Verification items for the finished model (mm, model axes). A direction names the side the tool comes from. Round coordinates to 2 decimals unless told otherwise and drop trailing zeros. Order: outer loops, then holes, each group sorted by start corner. A loop starts at its lowest first (then second) coordinate and runs counter-clockwise, first axis right, second up. Notation, with made-up numbers: M 55.25,84 L 96.25,84 A14 cw 96.25,97 Z; hole C 9,20.25 d6. An arc over 180 degrees is marked long. Answer as a JSON object with one key per item and string values. Group by question number.
```python
from build123d import *

# Parameters (mm, degrees)
ESQUISSE1_R                  = 7.5
BOSS_EXTRU_1_DEPTH           = 10
ESQUISSE1_5_R                = 14
ENL_V_MAT_EXTRU_1_DEPTH      = 2
ENL_V_MAT_EXTRU_1_DEPTH_BACK = 10
BOSS_EXTRU_2_DEPTH           = 45
ENL_V_MAT_EXTRU_2_DEPTH      = 11
ENL_V_MAT_EXTRU_2_DEPTH_BACK = 21


with BuildPart() as part:
    # Esquisse1 → Boss.-Extru.1 (new body, symmetric)
    with BuildSketch(Plane.XY):
        with BuildLine():
            Line((-634.508066615, 20.5), (-595.008671928, 20.5))
            Line((-595.008671928, 20.5), (-595.008671928, -24.5))
            Line((-595.008671928, -24.5), (-634.508066615, -24.5))
            ThreePointArc((-634.508066615, -24.5), (-657.008066615, -2), (-634.508066615, 20.5))
        make_face()
        with Locations((-634.508066615, -2)):
            Circle(ESQUISSE1_R, mode=Mode.SUBTRACT)
    extrude(amount=BOSS_EXTRU_1_DEPTH, both=True)

    # Esquisse1_5 → Enl_v. mat.-Extru.1 (cut, two sides)
    with BuildSketch(Plane.XY) as enl_v_mat_extru_1_sk:
        with Locations((-634.508066615, -2)):
            Circle(ESQUISSE1_5_R)
    extrude(amount=ENL_V_MAT_EXTRU_1_DEPTH, mode=Mode.SUBTRACT)
    extrude(enl_v_mat_extru_1_sk.sketch, amount=-ENL_V_MAT_EXTRU_1_DEPTH_BACK, mode=Mode.SUBTRACT)

    # Esquisse2 → Boss.-Extru.2 (add)
    with BuildSketch(Plane(origin=(0, 20.5, 0), x_dir=(1, 0, 0), z_dir=(0, 1, 0))):
        Polygon((-605.008671928, 10), (-605.008671928, 15), (-600.008671928, 15), (-600.008671928, 20), (-620.008671928, 20), (-620.008671928, 15), (-615.008671928, 15), (-615.008671928, 10), align=None)
    extrude(amount=-BOSS_EXTRU_2_DEPTH)

    # Esquisse1_7 → Enl_v. mat.-Extru.2 (cut, two sides)
    with BuildSketch(Plane.XY) as enl_v_mat_extru_2_sk:
        Polygon((-612.508671928, -21.5), (-612.508671928, -24.5), (-607.508671928, -24.5), (-607.508671928, -21.5), (-606.008671928, -21.5), (-606.008671928, -18.5), (-614.008671928, -18.5), (-614.008671928, -21.5), align=None)
    extrude(amount=ENL_V_MAT_EXTRU_2_DEPTH, mode=Mode.SUBTRACT)
    extrude(enl_v_mat_extru_2_sk.sketch, amount=-ENL_V_MAT_EXTRU_2_DEPTH_BACK, mode=Mode.SUBTRACT)


solid = part.part
```
Q1. Cross-section at A-A, the plane y = -2. Record the cut outline in (x, z), then the cut area to 3 significant figures.
Q2. Thickness scan on line 1 (Z direction, x = -601, y = -8); line 2 (X direction, y = -2, z = 4.5); line 3 (Z direction, x = -648.5, y = 4). Record the ranges inside material, lowest first. Write a range as from..to.
Q3. Cross-section at D-D, the plane x = -618. Record the cut outline in (y, z).
Q4. Gauge pin test, flat ends, axial feed: pin 1 Ø19.5 at (x, y) = (-634.51, -2) entering from +Z; pin 2 Ø2.5 at (y, z) = (-20, -7) entering from -X; pin 3 Ø17 at (x, y) = (-634.51, -2) entering from -Z; pin 4 Ø12.5 at (x, y) = (-632.5, -11) entering from -Z. Record the tip position at first contact, or that the pin passes through.
Q5. Release check for a two-part mould opening along Y. For faces 6 (the face through (-628, -8, 2)), 7 (the face through (-600.009, -2, -17)), 8 (the face through (-657.003, -2.495, 0.14)) record: released by +Y, released by -Y, zero draft, split by the parting line, or undercut.
Q6. Tool access check on faces 1 (the face through (-623, -24.5, -1)), 2 (the face through (-615.009, -2, -13)), 3 (the face through (-605.009, -2, -12)), 4 (the face through (-626, -2, 10)), 5 (the face through (-620.009, -2, -18)). Record the directions out of +Z, -Z, +X, -X, +Y, -Y that give a thin tool (end or side, any length) a straight path to the whole face; none if there is none.
Q7. Cross-section at B-B, the plane z = 7. Record the cut outline in (x, y).
Q8. Cross-section at C-C, the plane x = -632.5. Record the cut outline in (y, z).
Conclusion:
{
 "1": {"outline": "M -657.01,-10 L -648.51,-10 L -648.51,2 L -642.01,2 L -642.01,10 L -657.01,10 Z; M -627.01,2 L -620.51,2 L -620.51,-10 L -615.01,-10 L -615.01,-15 L -620.01,-15 L -620.01,-20 L -600.01,-20 L -600.01,-15 L -605.01,-15 L -605.01,-10 L -595.01,-10 L -595.01,10 L -627.01,10 Z", "area": "934 mm2"},
 "2": {"line 1": "-20..-15, -10..10", "line 2": "-657.01..-642.01, -627.01..-595.01", "line 3": "-10..10"},
 "3": {"outline": "M -24.5,-20 L 20.5,-20 L 20.5,-15 L -24.5,-15 Z; M -24.5,-10 L 20.5,-10 L 20.5,10 L -24.5,10 Z"},
 "4": {"pin 1": "z = 10", "pin 2": "x = -649.53", "pin 3": "z = 2", "pin 4": "z = -10"},
 "5": {"face 6": "undercut", "face 7": "zero draft", "face 8": "split by the parting line"},
 "6": {"face 1": "+Z, -Z, +X, -X, -Y", "face 2": "-X, +Y, -Y", "face 3": "+X, +Y, -Y", "face 4": "+Z, +X, -X, +Y, -Y", "face 5": "-Z, -X, +Y, -Y"},
 "7": {"outline": "M -634.51,-24.5 L -612.51,-24.5 L -612.51,-21.5 L -614.01,-21.5 L -614.01,-18.5 L -606.01,-18.5 L -606.01,-21.5 L -607.51,-21.5 L -607.51,-24.5 L -595.01,-24.5 L -595.01,20.5 L -634.51,20.5 A22.5 ccw Z; hole C -634.51,-2 d15"},
 "8": {"outline": "M -24.5,-10 L -15.86,-10 L -15.86,2 L -9.23,2 L -9.23,10 L -24.5,10 Z; M 5.23,2 L 11.86,2 L 11.86,-10 L 20.5,-10 L 20.5,10 L 5.23,10 Z"}
}
